```python
from build123d import *


with BuildPart() as part:
    # Sketch1 → Revolve1 (revolve)
    with BuildSketch(Plane.XY, mode=Mode.PRIVATE) as revolve1_sk:
        with BuildLine():
            Line((0, 0), (0, 130))
            Line((0, 130), (16, 130))
            Line((16, 130), (16, 115))
            Line((16, 115), (14, 115))
            Line((14, 115), (14, 15))
            Line((14, 15), (16, 15))
            Line((16, 15), (17.111692668, 10.512431094))
            ThreePointArc((17.111692668, 10.512431094), (17.441933325, 9.984863822), (18.020263304, 9.754819144))
            Line((18.020263304, 9.754819144), (29.564485303, 9.036667386))
            add(Edge.make_bspline(
                [(29.564485303, 9.036667386), (30.853089791, 8.614064405), (31, 7.5)],
                knots=[0, 0, 0, 1, 1, 1], degree=2))
            add(Edge.make_bspline(
                [(29.564485303, 5.963332614), (30.853089791, 6.385935595), (31, 7.5)],
                knots=[0, 0, 0, 1, 1, 1], degree=2))
            Line((29.564485303, 5.963332614), (18.020263304, 5.245180856))
            ThreePointArc((18.020263304, 5.245180856), (17.441933325, 5.015136178), (17.111692668, 4.487568906))
            Line((17.111692668, 4.487568906), (16, 0))
            Line((16, 0), (0, 0))
        make_face()
    revolve(revolve1_sk.sketch.rotate(Axis((0, 0, 0), (0, 1, 0)), 90), axis=Axis((0, 0, 0), (0, 1, 0)))


solid = part.part
```
Geometry: final body of the model. Coordinates: model frame, mm. A direction names the side the tool comes from. Round coordinates to 2 decimals unless told otherwise and drop trailing zeros. Write each loop counter-clockwise with the first axis right and the second up, starting at its lowest first coordinate (ties: lowest second). Pieces come first, ordered by that corner, then holes. Notation, with made-up numbers: M 56.5,55 L 81.5,55 A32 ccw 81.5,82 Z; hole C -11,-17 d10. An arc over 180 degrees is marked long. Answer in a Markdown table with one row per item. Add a question column.
(1) Reachability of faces 1 (the face through (-15.67, 5.28, -9.99)), 2 (the face through (14.15, 115, 0.07)) from +Z, -Z, +X, -X, +Y, -Y: full face, straight path, thin tool, end or side. Return the list, or none.
(2) Cut plane A-A, the plane y = 83. Return the cut outline in (x, z), then the cut area to 3 significant figures.
(3) Ray query, L1, parallel to X at y = 82, z = -1.5; L2, parallel to Y at x = 25.5, z = 14; L3, parallel to Y at x = 4.5, z = -21. Return the intervals inside material, ascending.
(4) Draft query along Y for faces 3 (the face through (14.15, 15, -0.07)), 4 (the face through (15.62, 122.4, 3.47)), 5 (the face through (0, 0, 0)). Return one class per face: pulls with the +Y half, pulls with the -Y half, needs draft (parallel to the pull), parting line crosses it, or undercut.
(5) Contact query for flat-ended pins moving along their axis: pin 1 (8 mm diameter, centred on x = -8, y = 18.5, fed in from +Z); pin 2 (8 mm diameter, centred on x = 2.5, y = 70.5, fed in from +Z); pin 3 (3 mm diameter, centred on y = 44.5, z = 14, fed in from +X). Output: stop coordinate, or through.
Established:
| question | item | result |
|---|---|---|
| 1 | face 1 | -Y |
| 1 | face 2 | none |
| 2 | outline | C 0,0 d28 |
| 2 | area | 616 mm² |
| 3 | L1 | -13.92 to 13.92 |
| 3 | L2 | 5.93 to 9.07 |
| 3 | L3 | 5.46 to 9.54 |
| 4 | face 3 | undercut |
| 4 | face 4 | needs draft |
| 4 | face 5 | pulls with the -Y half |
| 5 | pin 1 | z = 14.81 |
| 5 | pin 2 | z = 14 |
| 5 | pin 3 | x = 6.3 |
